CAD build for the part. Positions are in the model's coordinates, mm. Round coordinates to 2 decimals unless told otherwise and drop trailing zeros. Write each loop counter-clockwise with the first axis right and the second up, starting at its lowest first coordinate (ties: lowest second). Pieces come first, ordered by that corner, then holes. Notation, with made-up numbers: (-28.5, -33) - (22.5, -33) arc R17 cw to (22.5, -14) - close; hole circle Ø2 at (64.5, 86). An arc over 180 degrees is marked (long way). Put each result on its own line as item: value. Start each with the question number.
Item 1: Cut at C-C (z = 2.3). Count the separate pieces of the cut face and the enclosed holes in it, and give its area (3 significant figures).
Item 2: Cut at A-A (x = -29.5). Give the cut face in (y, z).
Item 3: Drill centre lines: line 1 (X direction, y = 20, z = 2); line 2 (Y direction, x = 64, z = 2.8); line 3 (X direction, y = 108.5, z = 1.9). Where is each one in solid material? Low to high. Write a range as from..to.
Item 4: Cut at B-B (y = -48). Give the cut face in (x, z).
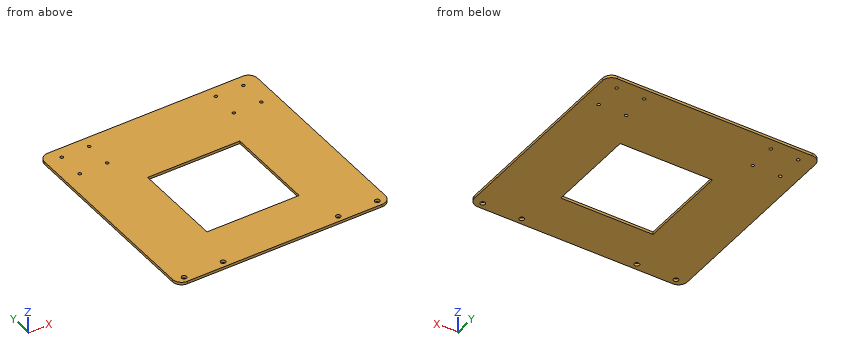
```python
from build123d import *

# Parameters (mm, degrees)
SKETCH3_R           = 1.75
SKETCH3_R_2         = 2.75
BOSS_EXTRUDE1_DEPTH = 3
SKETCH4_W           = 104
SKETCH4_H           = 102.1
CUT_EXTRUDE1_DEPTH  = 3


with BuildPart() as part:
    # Sketch3 → Boss-Extrude1 (new body)
    with BuildSketch(Plane.XY):
        with BuildLine():
            Line((118.968983292, -110.515508354), (118.968983292, 109.484491646))
            ThreePointArc((118.968983292, 109.484491646), (116.040051104, 116.555559458), (108.968983292, 119.484491646))
            Line((108.968983292, 119.484491646), (-111.031016708, 119.484491646))
            ThreePointArc((-111.031016708, 119.484491646), (-118.10208452, 116.555559458), (-121.031016708, 109.484491646))
            Line((-121.031016708, 109.484491646), (-121.031016708, -110.515508354))
            ThreePointArc((-121.031016708, -110.515508354), (-118.10208452, -117.586576166), (-111.031016708, -120.515508354))
            Line((-111.031016708, -120.515508354), (108.968983292, -120.515508354))
            ThreePointArc((108.968983292, -120.515508354), (116.040051104, -117.586576166), (118.968983292, -110.515508354))
        make_face()
        with Locations((-103.531016708, 75.984491646)):
            Circle(SKETCH3_R, mode=Mode.SUBTRACT)
        with Locations((-103.531016708, 106.984491646)):
            Circle(SKETCH3_R, mode=Mode.SUBTRACT)
        with Locations((-72.531016708, 106.984491646)):
            Circle(SKETCH3_R, mode=Mode.SUBTRACT)
        with Locations((-72.531016708, 75.984491646)):
            Circle(SKETCH3_R, mode=Mode.SUBTRACT)
        with Locations((-110.031016708, -113.515508354)):
            Circle(SKETCH3_R_2, mode=Mode.SUBTRACT)
        with Locations((-66.031016708, -113.515508354)):
            Circle(SKETCH3_R_2, mode=Mode.SUBTRACT)
        with Locations((63.968983292, -113.515508354)):
            Circle(SKETCH3_R_2, mode=Mode.SUBTRACT)
        with Locations((101.468983292, 75.984491646)):
            Circle(SKETCH3_R, mode=Mode.SUBTRACT)
        with Locations((101.468983292, 106.984491646)):
            Circle(SKETCH3_R, mode=Mode.SUBTRACT)
        with Locations((70.468983292, 106.984491646)):
            Circle(SKETCH3_R, mode=Mode.SUBTRACT)
        with Locations((70.468983292, 75.984491646)):
            Circle(SKETCH3_R, mode=Mode.SUBTRACT)
        with Locations((107.968983292, -113.515508354)):
            Circle(SKETCH3_R_2, mode=Mode.SUBTRACT)
    extrude(amount=BOSS_EXTRUDE1_DEPTH)

    # Sketch4 → Cut-Extrude1 (cut)
    with BuildSketch(Plane.XY.offset(3)):
        with Locations((-1.031016708, -14.965508354)):
            Rectangle(SKETCH4_W, SKETCH4_H)
    extrude(amount=-CUT_EXTRUDE1_DEPTH, mode=Mode.SUBTRACT)


solid = part.part
```
Output values:
1. separate pieces: 1
1. enclosed holes: 13
1. area: 46,700 mm2
2. outline: (-120.52, 0) - (-66.02, 0) - (-66.02, 3) - (-120.52, 3) - close; (36.08, 0) - (119.48, 0) - (119.48, 3) - (36.08, 3) - close
3. line 1: -121.03..-53.03, 50.97..118.97
3. line 2: -120.52..-116.27, -110.77..119.48
3. line 3: -121.03..-104.41, -102.66..-73.41, -71.66..69.59, 71.34..100.59, 102.34..118.97
4. outline: (-121.03, 0) - (-53.03, 0) - (-53.03, 3) - (-121.03, 3) - close; (50.97, 0) - (118.97, 0) - (118.97, 3) - (50.97, 3) - close
